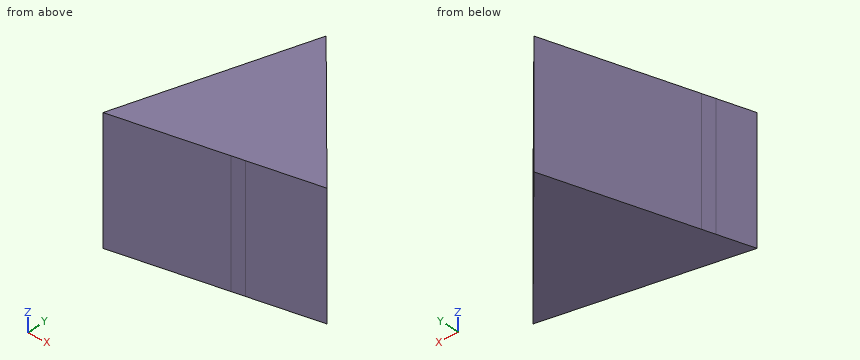
```python
from build123d import *

# Parameters (mm, degrees)
F1_DEPTH = 115.57


with BuildPart() as f1:
    # F0 (on Top) → F1 (new body)
    with BuildSketch(Plane.XY):
        Polygon((103.221436145, -53.8007080909), (-14.8500475308, 78.6029756424), (-56.6983165312, -48.1207240324), (-0.6158898202, 27.4022637386), (40.1904460134, -66.8826025271), align=None)
        Polygon((28.7687712922, -69.2531371272), (-60.2760904722, -58.9548340499), (-70.4792593606, -89.85177055), align=None)
        Polygon((-0.6158898202, 27.4022637386), (-56.6983165312, -48.1207240324), (-60.2760904722, -58.9548340499), (28.7687712922, -69.2531371272), (40.1904460134, -66.8826025271), align=None)
    extrude(amount=F1_DEPTH)


solid = f1.part
```
Design review of the part built by this model. Coordinates are the model's own, in mm. Give positions to 0.01 mm unless a question says otherwise; leave off trailing zeros. Write each loop counter-clockwise with the first axis right and the second up, starting at its lowest first coordinate (ties: lowest second). Pieces come first, ordered by that corner, then holes. Notation, with made-up numbers: (-18.5, 41) - (4.5, 41) arc R8 ccw to (4.5, 56) - close; hole circle Ø6 at (-32, 14.5). An arc over 180 degrees is marked (long way). Return JSON: item names as keys, results as strings. Group by question number.
(1) We need section C-C, the plane y = -44.5. Give the boundary of the cut face in (x, z), then the cut area to 3 significant figures.
(2) We need section A-A, the plane z = 18.5. Give the boundary of the cut face in (x, y).
(3) We need section B-B, the plane x = -28. Give the boundary of the cut face in (y, z).
(4) To check wall thickness, follow probe 1 along Y at (x, z) = (69, 59.5); probe 2 along Y at (x, z) = (3.5, 45.5); probe 3 along X at (y, z) = (33, 65). State the ranges of each line that lie inside material, in increasing order.
(5) Insertion check: pin 1 (1 mm diameter, centred on y = -50, z = 100.5, fed in from +X); pin 2 (8 mm diameter, centred on x = -31.5, z = 82, fed in from -Y); pin 3 (1 mm diameter, centred on x = 17, z = 42, fed in from +Y). Each pin has a flat end and moves straight along its axis. Give the tip position at first contact, or say it passes through.
Reported:
{
 "1": {"outline": "(-55.5, 0) - (94.93, 0) - (94.93, 115.57) - (-55.5, 115.57) - close", "area": "17,400 mm2"},
 "2": {"outline": "(-70.48, -89.85) - (103.22, -53.8) - (-14.85, 78.6) - close"},
 "3": {"outline": "(-81.04, 0) - (38.78, 0) - (38.78, 115.57) - (-81.04, 115.57) - close"},
 "4": {"probe 1": "y = -60.9 to -15.43", "probe 2": "y = -74.5 to 58.03", "probe 3": "x = -29.91 to 25.82"},
 "5": {"pin 1": "stops at x = 100.28", "pin 2": "stops at y = -82.59", "pin 3": "stops at y = 43.45"}
}
